```python
from build123d import *

# Parameters (mm, degrees)
SKETCH1_R                   = 60.7
BOSS_EXTRUDE1_DEPTH         = 1.5
M6_CLEARANCE_HOLE1_D        = 6.6
CIRPATTERN2_COUNT           = 4
SKETCH10_R                  = 7.5
SERVO_HUB_HOLE_DEPTH        = 86.895168665
SKETCH11_R                  = 2.25
SERVO_SCREW_HOLES_DEPTH     = 86.895168665
LEG_MECHANISM_CUTOUTS_DEPTH = 86.895168665
CIRPATTERN3_COUNT           = 4
M3_CLEARANCE_HOLE1_D        = 3.4


with BuildPart() as part:
    # Sketch1 → Boss-Extrude1 (new, symmetric)
    with BuildSketch(Plane(origin=(0, 0, 0), x_dir=(1, 0, 0), z_dir=(0, 1, 0))):
        with Locations(Location((0, 0, 0), (0, 0, 270))):
            Circle(SKETCH1_R)
    extrude(amount=BOSS_EXTRUDE1_DEPTH, both=True)

    # M6 Clearance Hole1 (through all)
    with Locations(Plane(origin=(0, 1.5, 0), x_dir=(1, 0, 0), z_dir=(0, 1, 0))):
        with Locations((50.7, 0)):
            m6_clearance_hole1 = Hole(M6_CLEARANCE_HOLE1_D / 2)

    # CirPattern2: M6 Clearance Hole1 ×4 about axis
    cirpattern2_axis = Axis((0, 0, 0), (0, 1, 0))
    for i in range(1, CIRPATTERN2_COUNT):
        add(m6_clearance_hole1.rotate(cirpattern2_axis, i * 360 / CIRPATTERN2_COUNT), mode=Mode.SUBTRACT)

    # Sketch10 → servo hub hole (cut, through all)
    with BuildSketch(Plane(origin=(0, 1.5, 0), x_dir=(1, 0, 0), z_dir=(0, 1, 0))):
        with Locations(Location((0, 0, 0), (0, 0, 270))):
            Circle(SKETCH10_R)
    extrude(amount=-SERVO_HUB_HOLE_DEPTH, mode=Mode.SUBTRACT)

    # Sketch11 → servo screw holes (cut, through all)
    with BuildSketch(Plane.XZ.offset(1.5)):
        with Locations(Location((-15.377499853, 2.468805027, 0), (0, 0, 270))):
            Circle(SKETCH11_R)
        with Locations(Location((-10.706440914, 11.310818846, 0), (0, 0, 270))):
            Circle(SKETCH11_R)
        with Locations(Location((28.390468552, -20.652936726, 0), (0, 0, 270))):
            Circle(SKETCH11_R)
        with Locations(Location((33.061527492, -11.810922906, 0), (0, 0, 270))):
            Circle(SKETCH11_R)
    extrude(amount=-SERVO_SCREW_HOLES_DEPTH, mode=Mode.SUBTRACT)

    # Sketch13 → leg mechanism cutouts (cut, through all)
    with BuildSketch(Plane(origin=(0, 1.5, 0), x_dir=(1, 0, 0), z_dir=(0, 1, 0))):
        with BuildLine():
            Line((31.677366544, -51.77870652), (20.273657909, -35.348386091))
            Line((20.273657909, -35.348386091), (26.024270059, -31.357088069))
            Line((26.024270059, -31.357088069), (37.427978694, -47.787408498))
            ThreePointArc((37.427978694, -47.787408498), (34.610255706, -49.8660225), (31.677366544, -51.77870652))
        make_face()
    leg_mechanism_cutouts = extrude(amount=-LEG_MECHANISM_CUTOUTS_DEPTH, mode=Mode.SUBTRACT)

    # CirPattern3: leg mechanism cutouts ×4 about axis
    cirpattern3_axis = Axis((0, 0, 0), (0, 1, 0))
    for i in range(1, CIRPATTERN3_COUNT):
        add(leg_mechanism_cutouts.rotate(cirpattern3_axis, i * 360 / CIRPATTERN3_COUNT), mode=Mode.SUBTRACT)

    # M3 Clearance Hole1 (through all)
    with Locations(Plane(origin=(0, 1.5, 0), x_dir=(1, 0, 0), z_dir=(0, 1, 0))):
        with Locations((8.604729668, 22.326187031), (10.204187746, 31.182920845)):
            Hole(M3_CLEARANCE_HOLE1_D / 2)


solid = part.part
```
The model under review builds one solid part; all positions refer to its coordinate system, in mm. A direction names the side the tool comes from. Coordinates: 2 decimals unless noted, no trailing zeros. Order: outer loops, then holes, each group sorted by start corner. A loop starts at its lowest first (then second) coordinate and runs counter-clockwise, first axis right, second up. Notation, with made-up numbers: M 74.25,35.5 L 132.25,35.5 A32 ccw 132.25,72.5 Z; hole C 70,81 d2. An arc over 180 degrees is marked long. One line per question, with ' | ' between items.
(1) Add section A-A, the plane x = 0. Write out the cut boundary in (y, z), then the cut area to 3 significant figures.
Geometry results:
outline: M -1.5,-60.7 L 1.5,-60.7 L 1.5,-54 L -1.5,-54 Z; M -1.5,-47.4 L 1.5,-47.4 L 1.5,-7.5 L -1.5,-7.5 Z; M -1.5,7.5 L 1.5,7.5 L 1.5,47.4 L -1.5,47.4 Z; M -1.5,54 L 1.5,54 L 1.5,60.7 L -1.5,60.7 Z | area: 280 mm²
(2) Add section C-C, the plane y = -0.1. State how many separate pieces and enclosed holes the cut face has, then the cut area to 3 significant figures.
Geometry results:
separate pieces: 1 | enclosed holes: 11 | area: 10,600 mm²
(3) Insertion check: pin 1 (6 mm diameter, centred on x = 0, z = -50.7, fed in from +Y); pin 2 (1.5 mm diameter, centred on x = 33, y = 0, fed in from +Z); pin 3 (1 mm diameter, centred on y = 0.5, z = -36, fed in from +X); pin 4 (1.5 mm diameter, centred on y = 0, z = 28.5, fed in from +X). Each pin has a flat end and moves straight along its axis. Give the tip position at first contact, or say it passes through.
Geometry results:
pin 1: passes through | pin 2: stops at z = 42.49 | pin 3: stops at x = 46.45 | pin 4: stops at x = 53.99
(4) Machinability: for faces 4 (the face through (-31.65, 0.02, -39.46)), 5 (the face through (59.62, 0.02, 11.4)), which of the approach directions +Z, -Z, +X, -X, +Y, -Y give a long, thin tool a straight path to every point of the face, cutting with its end or side? Answer none if there is none.
Geometry results:
face 4: +Y, -Y | face 5: +X, +Y, -Y
(5) Add section B-B, the plane z = -39.5. Write out the cut boundary in (x, y), then the cut area to 3 significant figures.
Geometry results:
outline: M -46.09,-1.5 L -31.68,-1.5 L -31.68,1.5 L -46.09,1.5 Z; M -23.16,-1.5 L 46.09,-1.5 L 46.09,1.5 L -23.16,1.5 Z | area: 251 mm²
(6) For probe 1 along Z at (x, y) = (-1, -0.75); probe 2 along Z at (x, y) = (32.5, -1); probe 3 along Z at (x, y) = (36, -0.15), list the stretches that pass through material, from the lowest coordinate up. Write a range as from..to.
Geometry results:
probe 1: z = -60.69..-53.84, -47.56..-7.43, 7.43..47.56, 53.84..60.69 | probe 2: z = -51.27..-26.82, -24.38..-13.99, -9.63..40.69 | probe 3: z = -48.87..-29.25, -20.73..45.73
(7) The part is to be moulded in two halves that separate along Z. For faces 1 (the face through (1, 1.5, 13)), 2 (the face through (-11.4, 0.02, 59.62)), 3 (the face through (29.066, -0.021, -22.799)), say which applies: +Z half, -Z half, draft (parallel to the pull), parting line (faces both ways), or undercut.
Geometry results:
face 1: draft | face 2: +Z half | face 3: undercut
